```python
from build123d import *

# Parameters (mm, degrees)
SKETCH2_R             = 76.2
SKETCH2_R_2           = 66.675
BOSS_EXTRUDE1_DEPTH   = 7.62
BOSS_EXTRUDE2_START   = 1.27
SKETCH2_3_R           = 66.675
SKETCH2_3_R_2         = 57.15
BOSS_EXTRUDE2_DEPTH   = 7.62
F_6_32_TAPPED_HOLE1_D = 2.7051
F_6_32_TAPPED_HOLE2_D = 2.7051


with BuildPart() as part:
    # Sketch2 → Boss-Extrude1 (new body)
    with BuildSketch(Plane.XY):
        with Locations(Location((0, 0, 0), (0, 0, 180))):
            Circle(SKETCH2_R)
        with Locations(Location((0, 0, 0), (0, 0, 180))):
            Circle(SKETCH2_R_2, mode=Mode.SUBTRACT)
    extrude(amount=BOSS_EXTRUDE1_DEPTH)

    # Sketch2_3 → Boss-Extrude2 (add)
    with BuildSketch(Plane.XY.offset(BOSS_EXTRUDE2_START)):
        with Locations(Location((0, 0, 0), (0, 0, 180))):
            Circle(SKETCH2_3_R)
        with Locations(Location((0, 0, 0), (0, 0, 180))):
            Circle(SKETCH2_3_R_2, mode=Mode.SUBTRACT)
    extrude(amount=BOSS_EXTRUDE2_DEPTH)

    # 6-32 Tapped Hole1 (through all)
    with Locations(Plane(origin=(-30.56255, 52.935889409, 8.89), x_dir=(1, 0, 0), z_dir=(0, 0, 1))):
        with Locations((0, 0), (-22.373339409, -22.373339409), (-30.56255, -52.935889409), (-22.373339409, -83.498439409), (0, -105.871778818), (30.56255, -114.060989409), (61.1251, -105.871778818), (83.498439409, -83.498439409), (91.68765, -52.935889409), (83.498439409, -22.373339409), (61.1251, 0), (30.56255, 8.189210591)):
            Hole(F_6_32_TAPPED_HOLE1_D / 2)

    # 6-32 Tapped Hole2 (through all)
    with Locations(Plane(origin=(0, 72.2376, 7.62), x_dir=(1, 0, 0), z_dir=(0, 0, 1))):
        with Locations((0, 0), (-36.1188, -9.678003292), (-62.559596708, -36.1188), (-72.2376, -72.2376), (-62.559596708, -108.3564), (-36.1188, -134.797196708), (0, -144.4752), (36.1188, -134.797196708), (62.559596708, -108.3564), (72.2376, -72.2376), (62.559596708, -36.1188), (36.1188, -9.678003292)):
            Hole(F_6_32_TAPPED_HOLE2_D / 2)


solid = part.part
```
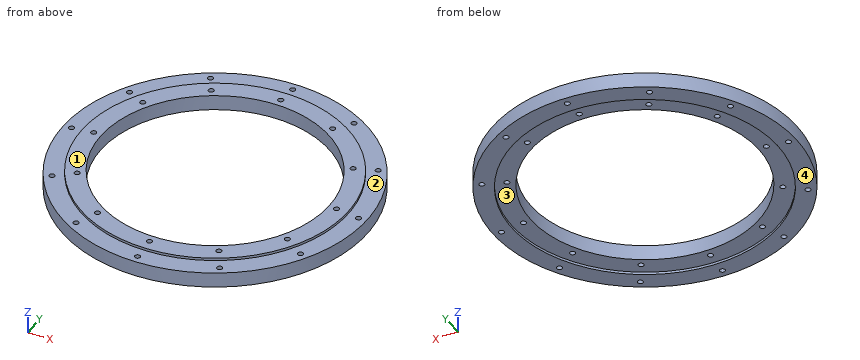
Input: part model. Units: mm. Frame: model coordinates. Face numbers are marked on the shaded views. A direction names the side the tool comes from. Coordinates: 2 decimals unless noted, no trailing zeros. Write each loop counter-clockwise with the first axis right and the second up, starting at its lowest first coordinate (ties: lowest second). Pieces come first, ordered by that corner, then holes.
1) Section C-C on y = -25.5. Output: boundary loops of the cut face in (x, z), and give its area (3 significant figures).
2) Section B-B on z = 5.25. State how many separate pieces and enclosed holes the cut face has, and give its area (3 significant figures).
3) Mould query, pull axis Y, two halves, no side actions, for the marked faces 3 and 4. Classes: pulls with the +Y half, pulls with the -Y half, needs draft (parallel to the pull), parting line crosses it, or undercut.
4) Section A-A on x = -24. Output: boundary loops of the cut face in (y, z), and give its area (3 significant figures).
5) Set-up query: the marked faces 1 and 2. Return all of +Z, -Z, +X, -X, +Y, -Y with unobstructed straight access to the full face (end or side cutting, diameter ignored); none if empty.
6) Material intervals for line 1 along Y through (x, z) = (0, 4); line 2 along X through (y, z) = (-30, 3), sorted ascending.
7) Pin query (flat end, axial travel): pin 1 Ø3 at (x, z) = (-36, 4.5) entering from +Y; pin 2 Ø3 at (x, y) = (-52.94, 30.56) entering from +Z; pin 3 Ø2 at (y, z) = (-4.5, 7) entering from +X; pin 4 Ø1.5 at (y, z) = (-20.5, 7) entering from -X. Return the tip coordinate at first contact, or that it passes through.
Check result:
1. outline: (-71.81, 0) - (-61.61, 0) - (-61.61, 1.27) - (-51.15, 1.27) - (-51.15, 8.89) - (-61.61, 8.89) - (-61.61, 7.62) - (-71.81, 7.62) - close; (51.15, 1.27) - (61.61, 1.27) - (61.61, 0) - (71.81, 0) - (71.81, 7.62) - (61.61, 7.62) - (61.61, 8.89) - (51.15, 8.89) - close
1. area: 315 mm2
2. separate pieces: 1
2. enclosed holes: 25
2. area: 7,840 mm2
3. face 3: undercut
3. face 4: needs draft
4. outline: (-72.32, 0) - (-62.21, 0) - (-62.21, 1.27) - (-51.87, 1.27) - (-51.87, 8.89) - (-62.21, 8.89) - (-62.21, 7.62) - (-72.32, 7.62) - close; (51.87, 1.27) - (62.21, 1.27) - (62.21, 0) - (72.32, 0) - (72.32, 7.62) - (62.21, 7.62) - (62.21, 8.89) - (51.87, 8.89) - close
4. area: 312 mm2
5. face 1: +Z, +X, -X, +Y, -Y
5. face 2: +Z
6. line 1: y = -76.2 to -73.59, -70.89 to -62.48, -59.77 to -57.15, 57.15 to 59.77, 62.48 to 70.89, 73.59 to 76.2
6. line 2: x = -70.05 to -54.17, -51.71 to -48.64, 48.64 to 51.71, 54.17 to 70.05
7. pin 1: stops at y = 67.94
7. pin 2: stops at z = 8.89
7. pin 3: stops at x = 76.12
7. pin 4: stops at x = -73.6
